Input: dimensioned drawing with shaded views. Units: mm. Origin: part minimum x, y, z. Coordinates: 2 decimals unless noted, no trailing zeros. Order: outer loops, then holes, each group sorted by start corner. A loop starts at its lowest first (then second) coordinate and runs counter-clockwise, first axis right, second up.
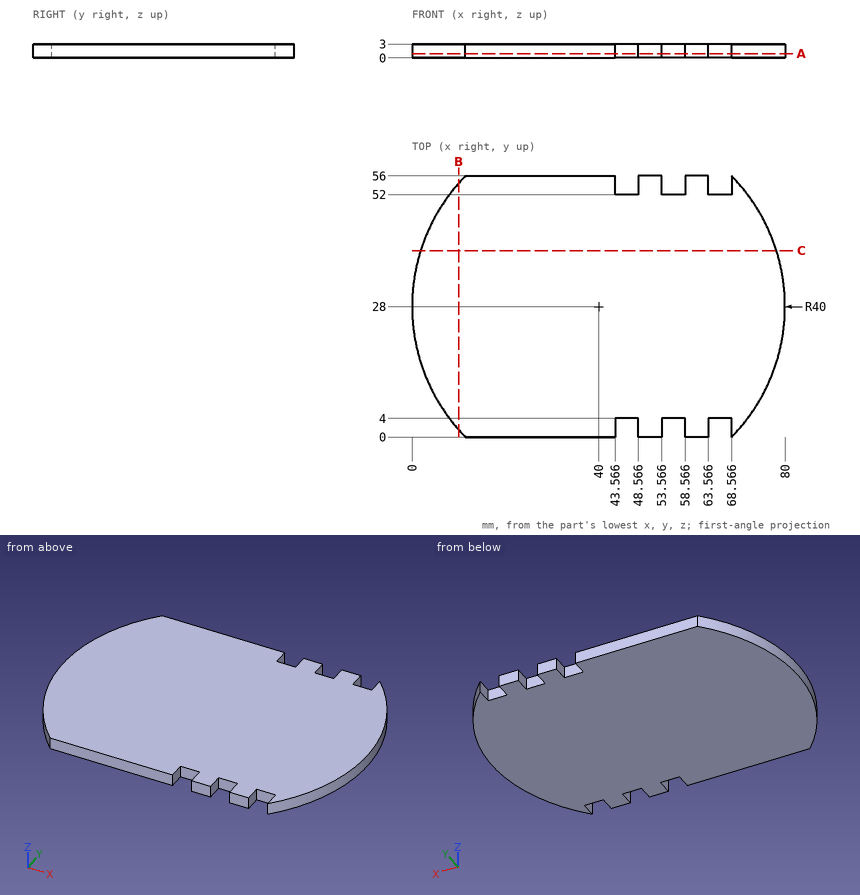
1. Section query C-C, the plane y = 40. Output: boundary loops of the cut face in (x, z), plus the area to 3 significant figures.
2. Contact query for flat-ended pins moving along their axis: P1, Ø1.5, axis at x = 55.5, z = 2, coming from the +Y side; P2, Ø1.5, axis at y = 1.5, z = 2, coming from the -X side; P3, Ø1.5, axis at y = 54, z = 1.5, coming from the +X side. Output: stop coordinate, or through.
3. Section query B-B, the plane x = 10. Output: boundary loops of the cut face in (y, z), plus the area to 3 significant figures.
4. Material intervals for line 1 along Y through (x, z) = (56.5, 2.25); line 2 along X through (y, z) = (3, 2.3) (1 decimal); line 3 along X through (y, z) = (2.5, 1.75) (1 decimal), sorted ascending.
5. Section query A-A, the plane z = 0.95. Output: boundary loops of the cut face in (x, y).
Answer key:
1. outline: (1.84, 0) - (78.16, 0) - (78.16, 3) - (1.84, 3) - close
1. area: 229 mm2
2. P1: stops at y = 52
2. P2: stops at x = 9.39
2. P3: stops at x = 71.02
3. outline: (1.54, 0) - (54.46, 0) - (54.46, 3) - (1.54, 3) - close
3. area: 159 mm2
4. line 1: y = 4 to 52
4. line 2: x = 8.8 to 43.6, 48.6 to 53.6, 58.6 to 63.6, 68.6 to 71.2
4. line 3: x = 9.2 to 43.6, 48.6 to 53.6, 58.6 to 63.6, 68.6 to 70.8
5. outline: (11.43, 0) - (43.57, 0) - (43.57, 4) - (48.57, 4) - (48.57, 0) - (53.57, 0) - (53.57, 4) - (58.57, 4) - (58.57, 0) - (63.57, 0) - (63.57, 4) - (68.57, 4) - (68.57, 0) arc R40 ccw to (68.57, 56) - (68.57, 52) - (63.57, 52) - (63.57, 56) - (58.57, 56) - (58.57, 52) - (53.57, 52) - (53.57, 56) - (48.57, 56) - (48.57, 52) - (43.57, 52) - (43.57, 56) - (11.43, 56) arc R40 ccw to start
